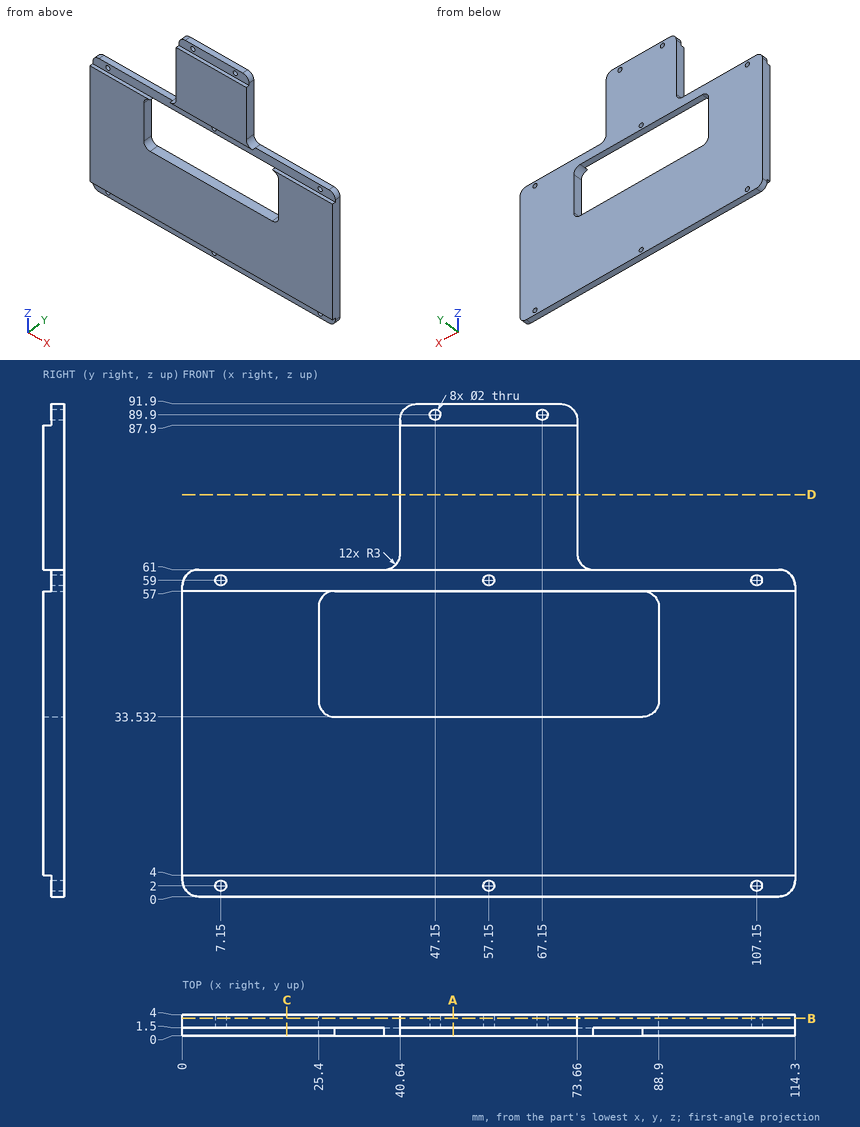
Can you work these out from the drawing? Everything is in mm from the part's minimum corner. Round coordinates to 2 decimals unless told otherwise and drop trailing zeros. Write each loop counter-clockwise with the first axis right and the second up, starting at its lowest first coordinate (ties: lowest second). Pieces come first, ordered by that corner, then holes. Notation, with made-up numbers: (74.25, -33) - (117.25, -33) arc R6 ccw to (117.25, -28) - close; hole circle Ø5 at (4, 69.25). An arc over 180 degrees is marked (long way). Put each result on its own line as item: value. Start each with the question number.
(1) I want a section at B-B, the plane y = 3.3. Give the number of separate pieces and of enclosed holes in the cut face, plus the area to 3 significant figures.
(2) I want a section at D-D, the plane z = 75. Please give me the cut outline in (x, y).
(3) I need wall thicknesses on probe 1 along Z at (x, y) = (107.15, 3.1); probe 2 along Z at (x, y) = (46, 3.45); probe 3 along Z at (x, y) = (67.15, 2.15). Which ranges of each line are inside material? Lowest first, please.
(4) I want a section at A-A, the plane x = 50.5. Please give me the cut outline in (y, z).
(5) Will these pins go through, and if not, where does the flat tip stop? pin 1 (2.5 mm diameter, centred on x = 47.15, z = 89.9, fed in from -Y); pin 2 (0.8 mm diameter, centred on x = 47.5, y = 3, fed in from -Z); pin 3 (0.8 mm diameter, centred on x = 60, y = 1, fed in from +Z); pin 4 (1.2 mm diameter, centred on y = 1.5, z = 77.5, fed in from +X).
(6) I want a section at C-C, the plane x = 19.5. Please give me the cut outline in (y, z), plus the area to 3 significant figures.
Here are the results:
1. separate pieces: 1
1. enclosed holes: 9
1. area: 6,480 mm^2
2. outline: (40.64, 0) - (73.66, 0) - (73.66, 4) - (40.64, 4) - close
3. probe 1: z = 0 to 1, 3 to 58, 60 to 61
3. probe 2: z = 0 to 33.53, 57 to 91.9
3. probe 3: z = 0 to 33.53, 57 to 88.9, 90.9 to 91.9
4. outline: (0, 4) - (1.5, 4) - (1.5, 0) - (4, 0) - (4, 33.53) - (0, 33.53) - close; (0, 61) - (1.5, 61) - (1.5, 57) - (4, 57) - (4, 91.9) - (1.5, 91.9) - (1.5, 87.9) - (0, 87.9) - close
5. pin 1: stops at y = 1.5
5. pin 2: stops at z = 0
5. pin 3: stops at z = 87.9
5. pin 4: stops at x = 73.66
6. outline: (0, 4) - (1.5, 4) - (1.5, 0) - (4, 0) - (4, 61) - (1.5, 61) - (1.5, 57) - (0, 57) - close
6. area: 232 mm^2
